```python
from build123d import *

# Parameters (mm, degrees)
F0_W     = 40
F0_H     = 40
F0_W_2   = 35
F0_H_2   = 35
F1_DEPTH = 100
F3_DEPTH = 40.001
F4_DEPTH = 40
F5_R     = 4
F6_DEPTH = 2.5
F8_DEPTH = 2.5
F9_R     = 5


with BuildPart() as f1:
    # F0 (on Top) → F1 (new body)
    with BuildSketch(Plane.XY):
        Rectangle(F0_W, F0_H)
        Rectangle(F0_W_2, F0_H_2, mode=Mode.SUBTRACT)
    extrude(amount=F1_DEPTH)

    # F2 (on face) → F3 (cut, through all)
    with BuildSketch(Plane.YZ.offset(20)):
        with BuildLine():
            Line((20, 25.3402171373), (20, 75.7902171373))
            ThreePointArc((20, 75.7902171373), (-5.225, 50.5652171373), (20, 25.3402171373))
        make_face()
        with BuildLine():
            ThreePointArc((20, 25.3402171373), (-5.225, 50.5652171373), (20, 75.7902171373))
            Line((20, 75.7902171373), (20, 78.7902171373))
            ThreePointArc((20, 78.7902171373), (-8.225, 50.5652171373), (20, 22.3402171373))
            Line((20, 22.3402171373), (20, 25.3402171373))
        make_face()
        Polygon((20, 0), (20, 12.3402171373), (-20, 30.5652171373), (-20, 0), align=None)
        Polygon((-20, 70.5652171373), (20, 88.7902171373), (20, 100), (-20, 100), align=None)
    extrude(amount=-F3_DEPTH, mode=Mode.SUBTRACT)

    # F2 (on face) → F4 (join)
    with BuildSketch(Plane.YZ.offset(20)):
        with BuildLine():
            ThreePointArc((20, 25.3402171373), (-5.225, 50.5652171373), (20, 75.7902171373))
            Line((20, 75.7902171373), (20, 78.7902171373))
            ThreePointArc((20, 78.7902171373), (-8.225, 50.5652171373), (20, 22.3402171373))
            Line((20, 22.3402171373), (20, 25.3402171373))
        make_face()
    extrude(amount=-F4_DEPTH)

    # F5 (on face) → F6 (cut)
    with BuildSketch(Plane(origin=(0, 20, 0), x_dir=(-1, 0, 0), z_dir=(0, 1, 0))):
        with Locations((0, 82.2902171373)):
            Circle(F5_R)
    extrude(amount=-F6_DEPTH, mode=Mode.SUBTRACT)

    # F7 (on face) → F8 (cut)
    with BuildSketch(Plane(origin=(0, 20, 0), x_dir=(-1, 0, 0), z_dir=(0, 1, 0))):
        with BuildLine():
            ThreePointArc((0, 22.8402171373), (-4, 18.8402171373), (0, 14.8402171373))
            Line((0, 14.8402171373), (0, 22.8402171373))
        make_face()
        with BuildLine():
            Line((0, 22.8402171373), (0, 14.8402171373))
            ThreePointArc((0, 14.8402171373), (2.8284271247, 16.0117900126), (4, 18.8402171373))
            ThreePointArc((4, 18.8402171373), (2.8284271247, 21.6686442621), (0, 22.8402171373))
        make_face()
    extrude(amount=-F8_DEPTH, mode=Mode.SUBTRACT)

    # F9
    f9_edges = [f1.edges().sort_by_distance(p)[0] for p in [
        (-20, 20, 82.290217),
        (-20, 20, 18.840217),
        (-20, -20, 50.565217),
        (20, -20, 50.565217),
        (20, 20, 18.840217),
        (20, 20, 82.290217),
    ]]
    fillet(f9_edges, radius=F9_R)


solid = f1.part
```
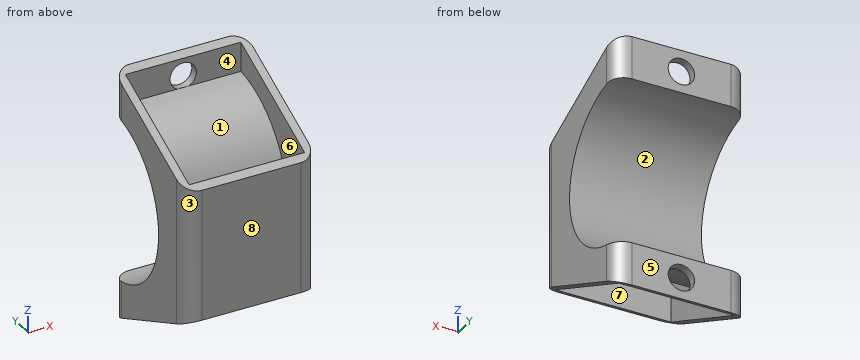
CAD build for the part. Positions are in the model's coordinates, mm. Face numbers are marked on the shaded views. A direction names the side the tool comes from. Give positions to 0.01 mm unless a question says otherwise; leave off trailing zeros. Order: outer loops, then holes, each group sorted by start corner. A loop starts at its lowest first (then second) coordinate and runs counter-clockwise, first axis right, second up. Notation, with made-up numbers: M 80,64 L 122,64 A25 ccw 122,76 Z; hole C 77.5,40 d3. An arc over 180 degrees is marked long. Put each result on its own line as item: value. Start each with the question number.
(1) Saw through at A-A, the plane x = 14. Write the cut outline in (y, z) (3 decimals), then the cut area to 3 significant figures.
(2) Saw through at C-C, the plane z = 56. Write the cut outline in (x, y), then the cut area to 3 significant figures.
(3) Mould opens along Y. For the marked faces 1, 2 and 3 say: +Y half, -Y half, draft (parallel to the pull), parting line (faces both ways), or undercut.
(4) Saw through at D-D, the plane y = 4. Write the cut outline in (x, z).
(5) Drill centre lines: line 1 along Z through (x, y) = (0, 19); line 2 along X through (y, z) = (-12, 49); line 3 along Z through (x, y) = (0, 18.5). Where is each one in solid material? Low to high.
(6) Flat gauge pins, fed straight in: pin 1 Ø3 at (x, y) = (-0.5, 8.5) entering from -Z; pin 2 Ø4.5 at (x, z) = (-3.5, 16) entering from -Y; pin 3 Ø5 at (y, z) = (5, 32) entering from +X; pin 4 Ø2 at (x, y) = (-9, -4) entering from +Z. Where does each tip first touch, or does it go through?
(7) Which spindle directions (+Z, -Z, +X, -X, +Y, -Y) get a long thin tool onto all of the face, cutting with end or side? Do the marked faces 4, 5, 6, 7 and 8. Say none if no direction does.
(8) Saw through at B-B, the plane y = 9. Write the cut outline in (x, z).
Check result:
1. outline: M -20,30.565 L -17.5,29.426 L -17.5,71.704 L -20,70.565 Z; M 17.5,13.479 L 20,12.34 L 20,25.34 A25.225 cw 20,75.79 L 20,88.79 L 17.5,87.651 L 17.5,78.679 A28.225 ccw 17.5,22.451 Z
1. area: 402 mm2
2. outline: M -20,-15 A5 ccw -15,-20 L 15,-20 A5 ccw 20,-15 L 20,-4.63 L -20,-4.63 Z; hole M -17.5,-17.5 L 17.5,-17.5 L 17.5,-7.7 L -17.5,-7.7 Z
2. area: 261 mm2
3. face 1: undercut
3. face 2: +Y half
3. face 3: -Y half
4. outline: M -20,19.63 L -17.5,19.63 L -17.5,27.31 L 17.5,27.31 L 17.5,19.63 L 20,19.63 L 20,31.06 L -20,31.06 Z; M -20,70.07 L 20,70.07 L 20,81.5 L 17.5,81.5 L 17.5,73.82 L -17.5,73.82 L -17.5,81.5 L -20,81.5 Z
5. line 1: z = 12.8 to 14.84, 22.84 to 25.36, 75.77 to 78.29, 86.29 to 88.33
5. line 2: x = -20 to -17.5, 17.5 to 20
5. line 3: z = 13.02 to 14.84, 22.84 to 25.38, 75.75 to 78.29, 86.29 to 88.11
6. pin 1: stops at z = 24.17
6. pin 2: stops at y = 17.5
6. pin 3: stops at x = 20
6. pin 4: stops at z = 66.93
7. face 4: +Z, -Y
7. face 5: +Z, -Z, +X, -X, +Y
7. face 6: none
7. face 7: +Z, -Z
7. face 8: +Z, -Z, +X, -X, -Y
8. outline: M -20,17.35 L -17.5,17.35 L -17.5,24.57 L 17.5,24.57 L 17.5,17.35 L 20,17.35 L 20,27.86 L -20,27.86 Z; M -20,73.27 L 20,73.27 L 20,83.78 L 17.5,83.78 L 17.5,76.56 L -17.5,76.56 L -17.5,83.78 L -20,83.78 Z
